For this review, use the dimensioned drawing (mm, ordinates from the lowest corner) and the shaded views. A direction names the side the tool comes from. Round coordinates to 2 decimals unless told otherwise and drop trailing zeros. Loops run counter-clockwise (first coordinate to the right, second up) from the corner with the lowest first, then second, coordinate; pieces in that order, holes last. Notation, with made-up numbers: M 7,-14.75 L 48,-14.75 A26 ccw 48,11.25 Z; hole C 84,37 d2. An arc over 180 degrees is marked long. Write item = value, one per line. Start each with the question number.
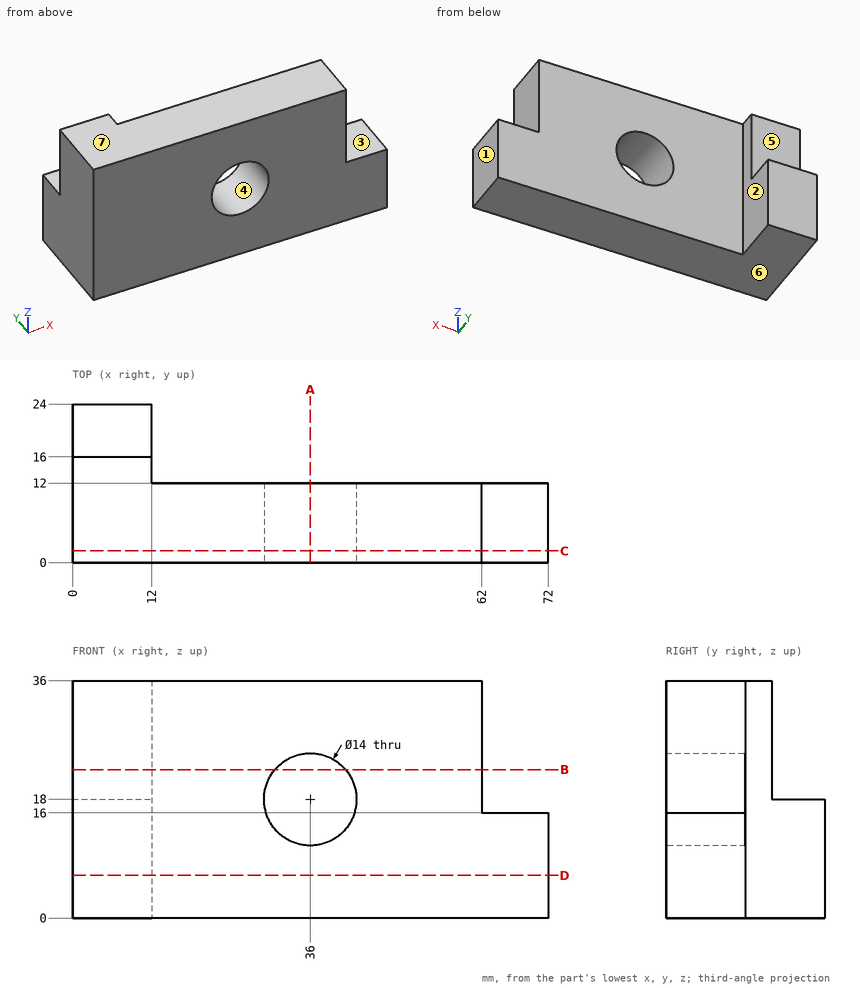
(1) Add section A-A on x = 36. Write out the cut boundary in (y, z), and give its area (3 significant figures).
(2) Tool access review of the marked faces 1, 2 and 3: name each direction out of +Z, -Z, +X, -X, +Y, -Y from which nothing blocks a thin tool from reaching the whole face with its end or side.
(3) Add section D-D on z = 6.5. Write out the cut boundary in (x, y), and give its area (3 significant figures).
(4) Draft analysis for pull direction Z (two halves, no side actions). For the marked faces 4, 5, 6 and 7, state which applies: +Z half, -Z half, draft (parallel to the pull), parting line (faces both ways), or undercut.
(5) Wall thickness on L1, parallel to X at y = 7.75, z = 18; L2, parallel to Y at x = 51.5, z = 14: over which ranges is each line inside the solid? List them lowest first.
(6) Add section B-B on z = 22.5. Write out the cut boundary in (x, y).
(7) For pin 1 Ø9.5 at (y, z) = (17, 23) entering from +X; pin 2 Ø2 at (x, z) = (11.5, 27.5) entering from +Y; pin 3 Ø6 at (x, z) = (63, 24.5) entering from -Y; pin 4 Ø3 at (x, y) = (68, 4) entering from +Z, all flat-tipped, find the tip position at first contact; note any pin that passes through.
(8) Add section C-C on y = 1.75. Write out the cut boundary in (x, z).
Answer sheet:
q1.outline = M 0,0 L 12,0 L 12,11 L 0,11 Z; M 0,25 L 12,25 L 12,36 L 0,36 Z
q1.area = 264 mm²
q2.face_1 = +Z, -Z, +X, +Y, -Y
q2.face_2 = +Z, -Z, +X, +Y
q2.face_3 = +Z, +X, +Y, -Y
q3.outline = M 0,0 L 72,0 L 72,12 L 12,12 L 12,24 L 0,24 Z
q3.area = 1,010 mm²
q4.face_4 = undercut
q4.face_5 = draft
q4.face_6 = -Z half
q4.face_7 = +Z half
q5.L1 = 0 to 29, 43 to 62
q5.L2 = 0 to 12
q6.outline = M 0,0 L 30.64,0 L 30.64,12 L 12,12 L 12,16 L 0,16 Z; M 41.36,0 L 62,0 L 62,12 L 41.36,12 Z
q7.pin_1 = 12
q7.pin_2 = 16
q7.pin_3 = 0
q7.pin_4 = 16
q8.outline = M 0,0 L 72,0 L 72,16 L 62,16 L 62,36 L 0,36 Z; hole C 36,18 d14
